```python
from build123d import *

# Parameters (mm, degrees)
SKETCH1_W           = 16
SKETCH1_H           = 16
SKETCH1_W_2         = 12
SKETCH1_H_2         = 12
BOSS_EXTRUDE1_DEPTH = 600
FILLET1_R           = 1
SKETCH2_R           = 2.5
CUT_EXTRUDE1_DEPTH  = 16
SKETCH3_R           = 2.5
CUT_EXTRUDE2_DEPTH  = 16


with BuildPart() as part:
    # Sketch1 → Boss-Extrude1 (new body)
    with BuildSketch(Plane(origin=(0, 0, 0), x_dir=(1, 0, 0), z_dir=(0, 1, 0))):
        with Locations((3.278287462, -2.788990826)):
            Rectangle(SKETCH1_W, SKETCH1_H)
        with Locations((3.278287462, -2.788990826)):
            Rectangle(SKETCH1_W_2, SKETCH1_H_2, mode=Mode.SUBTRACT)
    extrude(amount=BOSS_EXTRUDE1_DEPTH)

    # Fillet1
    fillet1_edges = [part.edges().sort_by_distance(p)[0] for p in [
        (-4.721712538, 300, -5.211009174),
        (11.278287462, 300, -5.211009174),
        (11.278287462, 300, 10.788990826),
        (-4.721712538, 300, 10.788990826),
    ]]
    fillet(fillet1_edges, radius=FILLET1_R)

    # Sketch2 → Cut-Extrude1 (cut)
    with BuildSketch(Plane.XY.offset(10.788990826)):
        with Locations((3.278287462, 592)):
            Circle(SKETCH2_R)
        with Locations((3.278287462, 8)):
            Circle(SKETCH2_R)
    extrude(amount=-CUT_EXTRUDE1_DEPTH, mode=Mode.SUBTRACT)

    # Sketch3 → Cut-Extrude2 (cut)
    with BuildSketch(Plane(origin=(11.278287462, 0, 0), x_dir=(0, 0, -1), z_dir=(1, 0, 0))):
        with Locations((-2.788990826, 450)):
            Circle(SKETCH3_R)
    extrude(amount=-CUT_EXTRUDE2_DEPTH, mode=Mode.SUBTRACT)


solid = part.part
```
Could you check a few things on this model? Use its own coordinates, in mm. A direction names the side the tool comes from. Give positions to 0.01 mm unless a question says otherwise; leave off trailing zeros. Loops run counter-clockwise (first coordinate to the right, second up) from the corner with the lowest first, then second, coordinate; pieces in that order, holes last. Notation, with made-up numbers: (17, 15) -> (44, 15) arc R23 cw to (44, 34) -> close; hole circle Ø8 at (74, 50). An arc over 180 degrees is marked (long way). Put each result on its own line as item: value.
(1) Thinking about a two-plate mould opening in X: for faces 3 (the face through (-4, 600, 3)), 4 (the face through (9.278, 296, 3)), 5 (the face through (11.278, 296, 3)), which applies, pulls with the +X half, pulls with the -X half, needs draft (parallel to the pull), parting line crosses it, or undercut?
Computed:
face 3: needs draft
face 4: undercut
face 5: pulls with the +X half
(2) Imagine slicing it at A-A on y = 560.5. Write out the boundary of the cut face in (x, z), plus the area to 3 significant figures.
Computed:
outline: (-4.72, -4.21) arc R1 ccw to (-3.72, -5.21) -> (10.28, -5.21) arc R1 ccw to (11.28, -4.21) -> (11.28, 9.79) arc R1 ccw to (10.28, 10.79) -> (-3.72, 10.79) arc R1 ccw to (-4.72, 9.79) -> close; hole (-2.72, -3.21) -> (9.28, -3.21) -> (9.28, 8.79) -> (-2.72, 8.79) -> close
area: 111 mm^2
(3) I'm going to push a flat-ended pin straight in: pin 1 Ø8 at (y, z) = (450, 2.79) entering from -X. Where does the tip first touch, or does it pass through?
Computed:
pin 1: x = -4.72
(4) Please list where these lines run through material, in increasing order: probe 1 along Z at (x, y) = (6.5, 540.5); probe 2 along X at (y, z) = (238.5, 5.5); probe 3 along Z at (x, y) = (-3.45, 450). Write a range as [from, to].
Computed:
probe 1: [-5.21, -3.21], [8.79, 10.79]
probe 2: [-4.72, -2.72], [9.28, 11.28]
probe 3: [-5.21, 0.29], [5.29, 10.79]
(5) For faces 1 (the face through (3, 296, -5.211)), 2 (the face through (3, 296, -3.211)), which set-ups out of +Z, -Z, +X, -X, +Y, -Y let a thin tool reach every point of the face, with its end or its side?
Computed:
face 1: -Z, +X, -X, +Y, -Y
face 2: +Y, -Y
